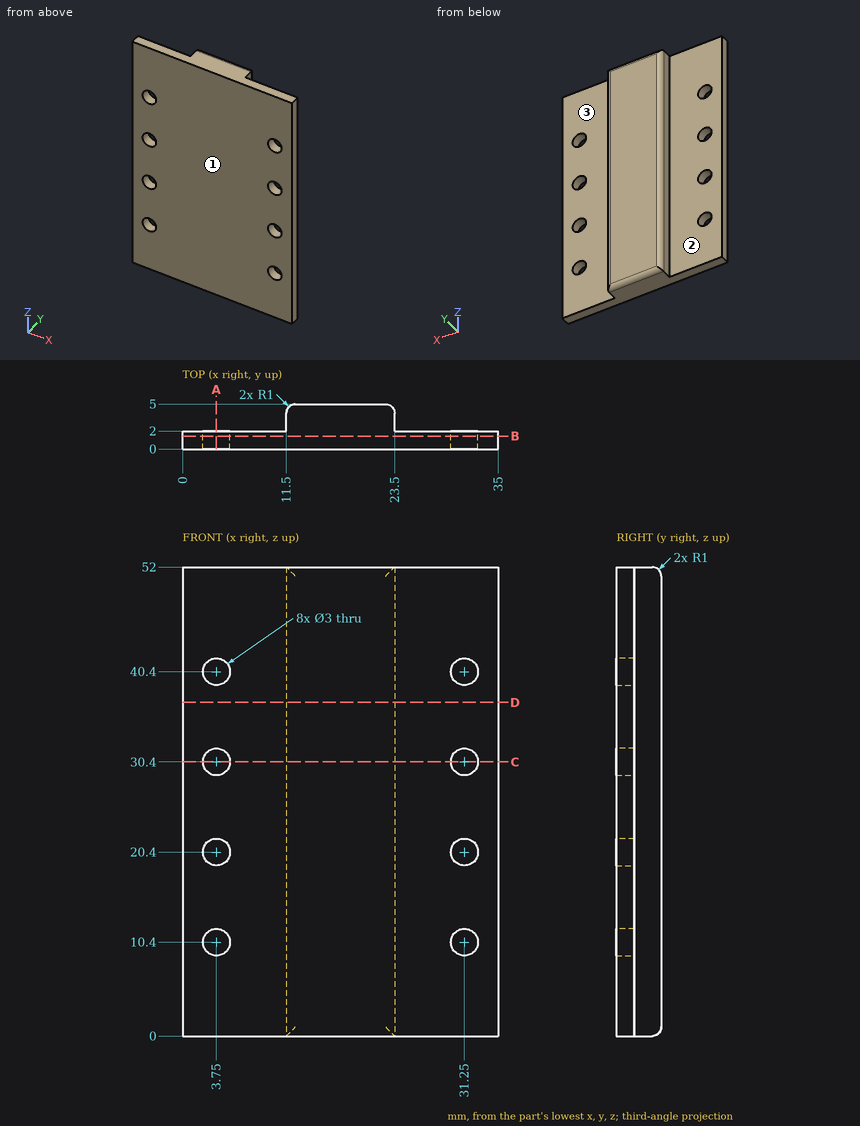
Job drawing, mm, ordinate dimensions from the low corner. One solid piece. A direction names the side the tool comes from. Coordinates: 2 decimals unless noted, no trailing zeros. Order: outer loops, then holes, each group sorted by start corner. A loop starts at its lowest first (then second) coordinate and runs counter-clockwise, first axis right, second up. Notation, with made-up numbers: (83.25, -1) -> (129.25, -1) arc R6 ccw to (129.25, 9) -> close; hole circle Ø2 at (57.25, 65.5). An arc over 180 degrees is marked (long way). Answer in a Markdown table with one row per item. Add a question column.
Q1. Drop flat-ended pins along their axis: pin 1 (2 mm diameter, centred on y = 4, z = 9, fed in from -X); pin 2 (0.6 mm diameter, centred on y = 2.5, z = 22.5, fed in from +X); pin 3 (6 mm diameter, centred on x = 31, z = 19.5, fed in from +Y); pin 4 (1.8 mm diameter, centred on x = 31.25, z = 10.4, fed in from -Y). Give the stop position or say it passes through.
Q2. Band-saw the part on B-B, the plane y = 1.45. Give the number of separate pieces and of enclosed holes in the cut face, then the cut area to 3 significant figures.
Q3. Band-saw the part on C-C, the plane z = 30.4. List the corners of the cut face in (x, y).
Q4. Band-saw the part on D-D, the plane z = 37. List the corners of the cut face in (x, y), then the cut area to 3 significant figures.
Q5. Wall check: line 1 along X through (y, z) = (0.45, 30.4); line 2 along Y through (x, z) = (11, 3.5); line 3 along X through (y, z) = (3.95, 35.5). Give the ranges that are in metal, low to high. Write a range as [from, to].
Q6. Band-saw the part on A-A, the plane x = 3.75. List the corners of the cut face in (y, z).
Q7. Which spindle directions (+Z, -Z, +X, -X, +Y, -Y) get a long thin tool onto all of the face, cutting with end or side? Do the marked faces 1, 2 and 3. Say none if no direction does.
Answers follow:
| question | item | result |
|---|---|---|
| 1 | pin 1 | x = 11.5 |
| 1 | pin 2 | x = 23.5 |
| 1 | pin 3 | y = 2 |
| 1 | pin 4 | through |
| 2 | separate pieces | 1 |
| 2 | enclosed holes | 8 |
| 2 | area | 1,760 mm^2 |
| 3 | outline | (0, 0) -> (2.25, 0) -> (2.25, 2) -> (0, 2) -> close; (5.25, 0) -> (29.75, 0) -> (29.75, 2) -> (23.5, 2) -> (23.5, 4) arc R1 ccw to (22.5, 5) -> (12.5, 5) arc R1 ccw to (11.5, 4) -> (11.5, 2) -> (5.25, 2) -> close; (32.75, 0) -> (35, 0) -> (35, 2) -> (32.75, 2) -> close |
| 4 | outline | (0, 0) -> (35, 0) -> (35, 2) -> (23.5, 2) -> (23.5, 4) arc R1 ccw to (22.5, 5) -> (12.5, 5) arc R1 ccw to (11.5, 4) -> (11.5, 2) -> (0, 2) -> close |
| 4 | area | 106 mm^2 |
| 5 | line 1 | [0, 2.25], [5.25, 29.75], [32.75, 35] |
| 5 | line 2 | [0, 2] |
| 5 | line 3 | [11.5, 23.5] |
| 6 | outline | (0, 0) -> (2, 0) -> (2, 8.9) -> (0, 8.9) -> close; (0, 11.9) -> (2, 11.9) -> (2, 18.9) -> (0, 18.9) -> close; (0, 21.9) -> (2, 21.9) -> (2, 28.9) -> (0, 28.9) -> close; (0, 31.9) -> (2, 31.9) -> (2, 38.9) -> (0, 38.9) -> close; (0, 41.9) -> (2, 41.9) -> (2, 52) -> (0, 52) -> close |
| 7 | face 1 | +Z, -Z, +X, -X, -Y |
| 7 | face 2 | +Z, -Z, -X, +Y |
| 7 | face 3 | +Z, -Z, +X, +Y |
